Autodesk Inventor part; units mm, degrees
ref_plane "YZ Plane" through (0, 0, 0) normal (1, 0, 0) x (0, 1, 0)
ref_plane "XZ Plane" through (0, 0, 0) normal (0, 1, 0) x (-1, 0, 0)
ref_plane "XY Plane" through (0, 0, 0) normal (0, 0, 1) x (1, 0, 0)
sketch "TopBoxFrame" plane through (0, 0, 0) normal (0, 0, 1) x (1, 0, 0)
  line L0 (0, 0) -> (292.1, 0)
  line L1 (292.1, 0) -> (292.1, 76.2)
  line L2 (292.1, 76.2) -> (0, 76.2)
  line L3 (0, 76.2) -> (0, 0)
  dimension "d3" = 76.2
  dimension "d27" = 292.1
extrude "TopBoxWidth" add sketch "TopBoxFrame" against normal blind 209.55
sketch "TrayShape" plane through (0, 0, 0) normal (0, 0, 1) x (1, 0, 0)
  line L0 (12.7, 63.5) -> (279.4, 63.5)
  line L1 (279.4, 63.5) -> (279.4, 0)
  line L2 (279.4, 0) -> (12.7, 0)
  line L3 (12.7, 0) -> (12.7, 63.5)
  line L4 (292.1, 76.2) -> (0, 76.2)
  line L5 (0, 76.2) -> (0, 0)
  line L6 (292.1, 0) -> (292.1, 76.2)
  line L7 (0, 0) -> (292.1, 0)
  dimension "d4" = 12.7
  dimension "d5" = 12.7
  dimension "d6" = 12.7
  dimension "d9" = 0
extrude "TrayCut" cut sketch "TrayShape" against normal blind 196.85 contours L0 L1 L2 L3
sketch "HoleGeometry" plane through (0, 0, 0) normal (0, 0, 1) x (1, 0, 0)
  line L0 (292.1, 0) -> (292.1, 76.2)
  line L1 (279.4, 63.5) -> (279.4, 0)
  line L2 (279.4, 0) -> (292.1, 0)
  line L3 (292.1, 0) -> (292.1, 76.2)
  line L4 (292.1, 76.2) -> (0, 76.2)
  line L5 (0, 76.2) -> (0, 0)
  line L6 (0, 0) -> (12.7, 0)
  line L7 (12.7, 0) -> (12.7, 63.5)
  line L8 (12.7, 63.5) -> (279.4, 63.5)
  line L9 (292.1, 76.2) -> (292.1, 0)
  line L10 (292.1, 0) -> (0, 0)
  line L11 (0, 0) -> (0, 76.2)
  line L12 (0, 76.2) -> (292.1, 76.2)
  point P0 (273.05, 69.85)
  point P1 (247.65, 69.85)
  point P2 (222.25, 69.85)
  point P3 (69.85, 69.85)
  point P4 (44.45, 69.85)
  point P5 (19.05, 69.85)
  dimension "d35" = 19.05
  dimension "d38" = 25.4
  dimension "d45" = 203.2
  dimension "d108" = 6.35
hole "FrontPlateHoles" at (273.05, 69.85, 0) at (247.65, 69.85, 0) at (222.25, 69.85, 0) at (69.85, 69.85, 0) at (44.45, 69.85, 0) at (19.05, 69.85, 0) direction (0, 0, -1) diameter 5.1054 depth 50.8 tip angle 118
sketch "BackHoleGeo" plane through (0, 0, -209.55) normal (0, 0, -1) x (-1, 0, 0)
  line L0 (-292.1, 76.2) -> (-292.1, 0)
  line L1 (-292.1, 0) -> (0, 0)
  line L2 (0, 0) -> (0, 76.2)
  line L3 (0, 76.2) -> (-292.1, 76.2)
  point P0 (-273.05, 69.85)
  point P1 (-247.65, 69.85)
  point P2 (-222.25, 69.85)
  point P3 (-69.85, 69.85)
  point P4 (-44.45, 69.85)
  point P5 (-19.05, 69.85)
  dimension "d57" = 19.05
  dimension "d60" = 25.4
  dimension "d67" = 203.2
  dimension "d107" = 6.35
hole "BackPlateHoles" at (273.05, 69.85, -209.55) at (247.65, 69.85, -209.55) at (222.25, 69.85, -209.55) at (69.85, 69.85, -209.55) at (44.45, 69.85, -209.55) at (19.05, 69.85, -209.55) direction (0, 0, 1) diameter 5.1054 depth 50.8 tip angle 118
sketch "RightHoleGeo" plane through (292.1, 0, 0) normal (1, 0, 0) x (0, 0, -1)
  line L0 (0, 76.2) -> (209.55, 76.2)
  line L1 (0, 0) -> (0, 76.2)
  line L2 (0, 0) -> (209.55, 0)
  point P0 (82.55, 6.35)
  point P1 (107.95, 6.35)
  point P2 (133.35, 6.35)
  dimension "d80" = 82.55
  dimension "d83" = 25.4
  dimension "d104" = 6.35
hole "RightPlateHoles" at (292.1, 6.35, -82.55) at (292.1, 6.35, -107.95) at (292.1, 6.35, -133.35) direction (-1, 0, 0) diameter 5.1054 depth 50.8 tip angle 118
sketch "LeftHoleGeo" plane through (0, 0, 0) normal (-1, 0, 0) x (0, 0, 1)
  line L0 (0, 76.2) -> (-209.55, 76.2)
  line L1 (-209.55, 0) -> (-209.55, 76.2)
  line L2 (0, 0) -> (-209.55, 0)
  point P0 (-127, 6.35)
  point P1 (-101.6, 6.35)
  point P2 (-76.2, 6.35)
  dimension "d96" = 82.55
  dimension "d99" = 25.4
  dimension "d105" = 6.35
hole "LeftPlateHoles" at (0, 6.35, -127) at (0, 6.35, -101.6) at (0, 6.35, -76.2) direction (1, 0, 0) diameter 5.1054 depth 50.8 tip angle 118
equation "\"d5\" = d4"
equation "\"d6\" = d5"
properties part number "BatteryBoxV2-Top"
CAD build for the part. Positions are in the model's coordinates, mm. A direction names the side the tool comes from. Coordinates: 2 decimals unless noted, no trailing zeros. Write each loop counter-clockwise with the first axis right and the second up, starting at its lowest first coordinate (ties: lowest second). Pieces come first, ordered by that corner, then holes.
(1) 3-axis set-ups, long thin cutter, end or side, ignore diameter. For faces 1 (the face through (145, 67, 0)), 2 (the face through (12.7, 31, -97)): which of +Z, -Z, +X, -X, +Y, -Y reach the whole face in a straight line?
(2) Drill centre lines: probe 1 along Z at (x, y) = (286.25, 6.35); probe 2 along X at (y, z) = (46, -194.5); probe 3 along Y at (x, z) = (5, -76.2). Where is each one in solid material? Low to high.
(3) Flat gauge pins, fed straight in: pin 1 (4.5 mm diameter, centred on y = 6.35, z = -133.35, fed in from +X); pin 2 (4 mm diameter, centred on x = 222.25, y = 69.85, fed in from -Z); pin 3 (3 mm diameter, centred on x = 44.45, y = 69.85, fed in from -Z). Where does each tip first touch, or does it go through?
(4) Cut at C-C, the plane z = -154. List the corners of the cut face in (x, y), and give its area (3 significant figures).
(5) Two-plate mould, pull along X, no slides. Class faces 3 (the face through (292.1, 38, -103)), 4 (the face through (144, 63.5, -97)), 5 (the face through (144, 39, -209.55)), 6 (the face through (0, 39, -103)): +X half, -X half, draft (parallel to the pull), parting line (faces both ways), or undercut.
(6) Cut at D-D, the plane x = 184. List the corners of the cut face in (y, z).
(7) Cut at A-A, the plane y = 44. List the corners of the cut face in (x, z).
(8) Cut at B-B, the plane z = -183. List the corners of the cut face in (x, y), and give its area (3 significant figures).
Geometry says:
1. face 1: +Z, +X, -X, +Y, -Y
1. face 2: +Z, -Y
2. probe 1: z = -209.55 to -135.9, -130.8 to -110.5, -105.4 to -85.1, -80 to 0
2. probe 2: x = 0 to 12.7, 279.4 to 292.1
2. probe 3: y = 0 to 3.8, 8.9 to 76.2
3. pin 1: stops at x = 12.7
3. pin 2: stops at z = -158.42
3. pin 3: stops at z = -158.12
4. outline: (0, 0) - (12.7, 0) - (12.7, 63.5) - (279.4, 63.5) - (279.4, 0) - (292.1, 0) - (292.1, 76.2) - (0, 76.2) - close
4. area: 5,320 mm2
5. face 3: +X half
5. face 4: undercut
5. face 5: draft
5. face 6: -X half
6. outline: (0, -209.55) - (76.2, -209.55) - (76.2, 0) - (63.5, 0) - (63.5, -196.85) - (0, -196.85) - close
7. outline: (0, -209.55) - (292.1, -209.55) - (292.1, 0) - (279.4, 0) - (279.4, -196.85) - (12.7, -196.85) - (12.7, 0) - (0, 0) - close
8. outline: (0, 0) - (12.7, 0) - (12.7, 63.5) - (279.4, 63.5) - (279.4, 0) - (292.1, 0) - (292.1, 76.2) - (0, 76.2) - close; hole circle Ø5.11 at (19.05, 69.85); hole circle Ø5.11 at (44.45, 69.85); hole circle Ø5.11 at (69.85, 69.85); hole circle Ø5.11 at (222.25, 69.85); hole circle Ø5.11 at (247.65, 69.85); hole circle Ø5.11 at (273.05, 69.85)
8. area: 5,200 mm2
